Geometry: final body of the model. Coordinates: model frame, mm. A direction names the side the tool comes from. Give positions to 0.01 mm unless a question says otherwise; leave off trailing zeros. Order: outer loops, then holes, each group sorted by start corner. A loop starts at its lowest first (then second) coordinate and runs counter-clockwise, first axis right, second up. Notation, with made-up numbers: (-11, 62.25) - (7, 62.25) arc R23 cw to (7, 76.25) - close; hole circle Ø9 at (44.5, 32.25). An arc over 180 degrees is marked (long way). Use one line per item in the form item = value.
from build123d import *

# Parameters (mm, degrees)
F0_W     = 203.2
F0_H     = 127
F1_DEPTH = 25.4
F2_W     = 50.8
F2_H     = 50.8
F3_DEPTH = 25.4
F4_R     = 25.4
F5_DEPTH = 25.401


with BuildPart() as f1:
    # F0 (on Top) → F1 (new body)
    with BuildSketch(Plane.XY):
        with Locations((101.6, 63.5)):
            Rectangle(F0_W, F0_H)
    extrude(amount=F1_DEPTH)

    # F2 (on face) → F3 (join)
    with BuildSketch(Plane.XY.offset(25.4)):
        with Locations((25.4, 25.4)):
            Rectangle(F2_W, F2_H)
        with Locations((177.8, 101.6)):
            Rectangle(F2_W, F2_H)
    extrude(amount=F3_DEPTH)

    # F4 (on face) → F5 (cut, through all)
    with BuildSketch(Plane.XY.offset(25.4)):
        with Locations((127, 50.8)):
            Circle(F4_R)
    extrude(amount=-F5_DEPTH, mode=Mode.SUBTRACT)


solid = f1.part
(1) Contact query for flat-ended pins moving along their axis: pin 1 Ø12.5 at (x, z) = (26.5, 41.5) entering from +Y; pin 2 Ø4 at (x, y) = (97.5, 72.5) entering from +Z; pin 3 Ø12.5 at (x, z) = (186.5, 35.5) entering from -Y. Output: stop coordinate, or through.
Computed values:
pin_1 = 50.8
pin_2 = 25.4
pin_3 = 76.2
(2) Cut plane B-B on z = 3. Output: boundary loops of the cut face in (x, y), plus the area to 3 significant figures.
Computed values:
outline = (0, 0) - (203.2, 0) - (203.2, 127) - (0, 127) - close; hole circle Ø50.8 at (127, 50.8)
area = 23,800 mm²
(3) Pull-direction query (Y, two-part tool) for faces 1 (the face through (140.65, 72.22, 12.88)), 2 (the face through (123, 127, 19)), 3 (the face through (177, 76.2, 38)), 4 (the face through (0, 48, 19)); classes: released by +Y, released by -Y, zero draft, split by the parting line, or undercut.
Computed values:
face_1 = undercut
face_2 = released by +Y
face_3 = released by -Y
face_4 = zero draft
(4) Ray query, line 1 along Y through (x, z) = (127, 6); line 2 along X through (y, z) = (50, 6); line 3 along X through (y, z) = (45.5, 8.5). Return the intervals inside material, ascending.
Computed values:
line_1 = 0 to 25.4, 76.2 to 127
line_2 = 0 to 101.61, 152.39 to 203.2
line_3 = 0 to 102.16, 151.84 to 203.2
(5) Cut plane A-A on x = 127. Output: boundary loops of the cut face in (y, z), plus the area to 3 significant figures.
Computed values:
outline = (0, 0) - (25.4, 0) - (25.4, 25.4) - (0, 25.4) - close; (76.2, 0) - (127, 0) - (127, 25.4) - (76.2, 25.4) - close
area = 1,940 mm²
(6) Cut plane D-D on x = 181. Output: boundary loops of the cut face in (y, z).
Computed values:
outline = (0, 0) - (127, 0) - (127, 50.8) - (76.2, 50.8) - (76.2, 25.4) - (0, 25.4) - close
(7) Cut plane C-C on y = 66. Output: boundary loops of the cut face in (x, z), plus the area to 3 significant figures.
Computed values:
outline = (0, 0) - (106.65, 0) - (106.65, 25.4) - (0, 25.4) - close; (147.35, 0) - (203.2, 0) - (203.2, 25.4) - (147.35, 25.4) - close
area = 4,130 mm²
(8) Reachability of faces 5 (the face through (203.2, 77, 19)), 6 (the face through (50.8, 25, 38)), 7 (the face through (25, 50.8, 38)), 8 (the face through (152.4, 101, 38)), 9 (the face through (100, 64, 0)) from +Z, -Z, +X, -X, +Y, -Y: full face, straight path, thin tool, end or side. Return the list, or none.
Computed values:
face_5 = +Z, -Z, +X, +Y, -Y
face_6 = +Z, +X, +Y, -Y
face_7 = +Z, +X, -X, +Y
face_8 = +Z, -X, +Y, -Y
face_9 = -Z, +X, -X, +Y, -Y
